For this review, take the finished solid that the model builds, in its own axes (mm). Face numbers are marked on the shaded views. A direction names the side the tool comes from. Give positions to 0.01 mm unless a question says otherwise; leave off trailing zeros. Write each loop counter-clockwise with the first axis right and the second up, starting at its lowest first coordinate (ties: lowest second). Pieces come first, ordered by that corner, then holes.
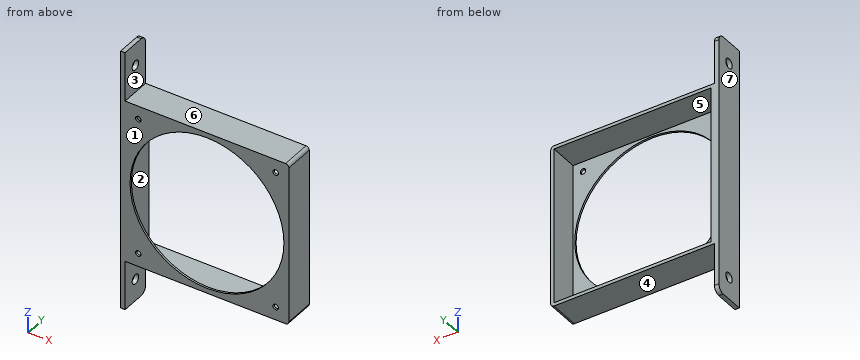
from build123d import *

# Parameters (mm, degrees)
SKETCH1_W           = 143
SKETCH1_H           = 143
BOSS_EXTRUDE1_DEPTH = 26
SKETCH2_R           = 70
SKETCH2_R_2         = 2.5
BOSS_EXTRUDE2_DEPTH = 1.8
SKETCH3_R           = 4.4
BOSS_EXTRUDE4_DEPTH = 4


with BuildPart() as part:
    # Sketch1 → Boss-Extrude1 (new body)
    with BuildSketch(Plane(origin=(0, 0, 0), x_dir=(1, 0, 0), z_dir=(0, 1, 0))):
        with BuildLine():
            Line((74.5, 71.5), (74.5, -71.5))
            ThreePointArc((74.5, -71.5), (73.621320344, -73.621320344), (71.5, -74.5))
            Line((71.5, -74.5), (-74.5, -74.5))
            Line((-74.5, -74.5), (-74.5, 74.5))
            Line((-74.5, 74.5), (71.5, 74.5))
            ThreePointArc((71.5, 74.5), (73.621320344, 73.621320344), (74.5, 71.5))
        make_face()
        Rectangle(SKETCH1_W, SKETCH1_H, mode=Mode.SUBTRACT)
    extrude(amount=BOSS_EXTRUDE1_DEPTH)

    # Sketch2 → Boss-Extrude2 (add)
    with BuildSketch(Plane.XZ):
        with BuildLine():
            Line((74.5, -71.5), (74.5, 71.5))
            ThreePointArc((74.5, 71.5), (73.621320344, 73.621320344), (71.5, 74.5))
            Line((71.5, 74.5), (-74.5, 74.5))
            Line((-74.5, 74.5), (-74.5, -74.5))
            Line((-74.5, -74.5), (71.5, -74.5))
            ThreePointArc((71.5, -74.5), (73.621320344, -73.621320344), (74.5, -71.5))
        make_face()
        with Locations(Location((0, 0, 0), (0, 0, 270))):
            Circle(SKETCH2_R, mode=Mode.SUBTRACT)
        with Locations(Location((-62.5, 62.5, 0), (0, 0, 270))):
            Circle(SKETCH2_R_2, mode=Mode.SUBTRACT)
        with Locations(Location((62.5, 62.5, 0), (0, 0, 270))):
            Circle(SKETCH2_R_2, mode=Mode.SUBTRACT)
        with Locations(Location((62.5, -62.5, 0), (0, 0, 270))):
            Circle(SKETCH2_R_2, mode=Mode.SUBTRACT)
        with Locations(Location((-62.5, -62.5, 0), (0, 0, 270))):
            Circle(SKETCH2_R_2, mode=Mode.SUBTRACT)
    extrude(amount=BOSS_EXTRUDE2_DEPTH)

    # Sketch3 → Boss-Extrude4 (add)
    with BuildSketch(Plane.ZY.offset(74.5)):
        with BuildLine():
            Line((-113.5, 26), (113.5, 26))
            ThreePointArc((113.5, 26), (117.742640687, 24.242640687), (119.5, 20))
            Line((119.5, 20), (119.5, -1.8))
            Line((119.5, -1.8), (-119.5, -1.8))
            Line((-119.5, -1.8), (-119.5, 20))
            ThreePointArc((-119.5, 20), (-117.742640687, 24.242640687), (-113.5, 26))
        make_face()
        with Locations((-99.5, 12.2)):
            Circle(SKETCH3_R, mode=Mode.SUBTRACT)
        with Locations((99.5, 12.2)):
            Circle(SKETCH3_R, mode=Mode.SUBTRACT)
    extrude(amount=BOSS_EXTRUDE4_DEPTH)


solid = part.part
(1) We need section C-C (x = 0). Write out the cut boundary in (y, z).
(2) Tool access review of the marked faces 4, 5, 6 and 7: name each direction out of +Z, -Z, +X, -X, +Y, -Y from which nothing blocks a thin tool from reaching the whole face with its end or side.
(3) We need section A-A (y = 12.2). Write out the cut boundary in (x, z).
(4) Clearance check with flat-ended pins moving along their axes: pin 1 Ø14 at (x, y) = (-15.5, 13.5) entering from -Z; pin 2 Ø4.5 at (x, z) = (62.5, -62.5) entering from +Y; pin 3 Ø6 at (x, z) = (-62.5, 62.5) entering from -Y; pin 4 Ø14 at (y, z) = (12.2, 99.5) entering from +X. State where each tip first meets the part, or that it passes through.
(5) We need section D-D (x = 62.5). Write out the cut boundary in (y, z), and give its area (3 significant figures).
(6) For L1, parallel to Y at x = -75.95, z = 99.5; L2, parallel to X at y = 16.25, z = -28; L3, parallel to Z at x = 44, y = 22.5, list the stretches that pass through material, from the lowest coordinate up.
(7) We need section B-B (z = -20.5). Write out the cut boundary in (x, y), and give its area (3 significant figures).
(8) The part is to be moulded in two halves that separate along X. For the marked faces 1, 2 and 3, say which applies: +X half, -X half, draft (parallel to the pull), parting line (faces both ways), or undercut.
The answers:
1. outline: (-1.8, -74.5) - (26, -74.5) - (26, -71.5) - (0, -71.5) - (0, -70) - (-1.8, -70) - close; (-1.8, 70) - (0, 70) - (0, 71.5) - (26, 71.5) - (26, 74.5) - (-1.8, 74.5) - close
2. face 4: -Z, +X, +Y, -Y
2. face 5: +Y
2. face 6: +Z, +X, +Y, -Y
2. face 7: +Z, -Z, -X, +Y, -Y
3. outline: (-78.5, -119.5) - (-74.5, -119.5) - (-74.5, -103.9) - (-78.5, -103.9) - close; (-78.5, -95.1) - (-74.5, -95.1) - (-74.5, -74.5) - (71.5, -74.5) arc R3 ccw to (74.5, -71.5) - (74.5, 71.5) arc R3 ccw to (71.5, 74.5) - (-74.5, 74.5) - (-74.5, 95.1) - (-78.5, 95.1) - close; (-78.5, 103.9) - (-74.5, 103.9) - (-74.5, 119.5) - (-78.5, 119.5) - close; hole (-71.5, -71.5) - (71.5, -71.5) - (71.5, 71.5) - (-71.5, 71.5) - close
4. pin 1: stops at z = -74.5
4. pin 2: passes through
4. pin 3: stops at y = -1.8
4. pin 4: stops at x = -74.5
5. outline: (-1.8, -74.5) - (26, -74.5) - (26, -71.5) - (0, -71.5) - (0, -65) - (-1.8, -65) - close; (-1.8, -60) - (0, -60) - (0, -31.52) - (-1.8, -31.52) - close; (-1.8, 31.52) - (0, 31.52) - (0, 60) - (-1.8, 60) - close; (-1.8, 65) - (0, 65) - (0, 71.5) - (26, 71.5) - (26, 74.5) - (-1.8, 74.5) - close
5. area: 293 mm2
6. L1: y = -1.8 to 7.8, 16.6 to 26
6. L2: x = -78.5 to -71.5, 71.5 to 74.5
6. L3: z = -74.5 to -71.5, 71.5 to 74.5
7. outline: (-78.5, -1.8) - (-66.93, -1.8) - (-66.93, 0) - (-71.5, 0) - (-71.5, 26) - (-78.5, 26) - close; (66.93, -1.8) - (74.5, -1.8) - (74.5, 26) - (71.5, 26) - (71.5, 0) - (66.93, 0) - close
7. area: 294 mm2
8. face 1: draft
8. face 2: undercut
8. face 3: +X half
